```python
from build123d import *

# Parameters (mm, degrees)
F1_DEPTH = 10
F2_T     = -1
F3_R     = 15.4445915984
F4_DEPTH = 25


with BuildPart() as f1:
    # F0 (on Top) → F1 (new body)
    with BuildSketch(Plane.XY):
        Polygon((-24.2622910139, -14.8777581411), (-53.029731502, -60.6361962855), (54.0178157389, -60.6361962855), (22.2354376062, -14.8777581411), (48.3378368161, -14.8777581411), (10.1295774803, 33.7235331535), (24.2622910139, 33.7235331535), (0, 68.0067832147), (-24.2622910139, 33.7235331535), (-8.3033312269, 33.7235331535), (-47.1593588355, -14.8777581411), align=None)
    extrude(amount=F1_DEPTH)

    # F2
    f2_openings = [f1.faces().sort_by_distance(p)[0] for p in [
        (0.198833, -13.317224, 10),
    ]]
    offset(amount=F2_T, openings=f2_openings, kind=Kind.INTERSECTION)

    # F3 (on face) → F4 (cut)
    with BuildSketch(Plane.XY.offset(1)):
        Circle(F3_R)
    extrude(amount=-F4_DEPTH, mode=Mode.SUBTRACT)


solid = f1.part
```
Check sheet for the modelled part. Datum: model origin and axes. Units: mm. A direction names the side the tool comes from. Round coordinates to 2 decimals unless told otherwise and drop trailing zeros. Order: outer loops, then holes, each group sorted by start corner. A loop starts at its lowest first (then second) coordinate and runs counter-clockwise, first axis right, second up. Notation, with made-up numbers: (-18, 87.25) - (26, 87.25) arc R25 ccw to (26, 121.25) - close; hole circle Ø11 at (25, 28). An arc over 180 degrees is marked (long way). Answer as CSV lines item,"result". Start each with the question number.
1) Depth check by flat-ended pin: pin 1 (1 mm diameter, centred on y = -44, z = 7, fed in from +X); pin 2 (18.5 mm diameter, centred on x = 0, y = 0, fed in from -Z); pin 3 (4.5 mm diameter, centred on x = 16.5, z = 6, fed in from +Y); pin 4 (1.5 mm diameter, centred on y = 2.5, z = 4, fed in from -X). Enter the tip coordinate at first touch or a pass-through.
2) Tool access check on faces 1 (the face through (-11.01, 50.72, 5.44)), 2 (the face through (-36, -14.878, 5)), 3 (the face through (38.35, -38.08, 4.93)), 4 (the face through (-11.96, 51.11, 4.93)). Record the directions out of +Z, -Z, +X, -X, +Y, -Y that give a thin tool (end or side, any length) a straight path to the whole face; none if there is none.
3) Section check A-A (z = 7.75). Record the cut outline in (x, y), then the cut area to 3 significant figures.
4) Section check B-B (x = -17.5). Record the cut outline in (y, z), then the cut area to 3 significant figures.
5) Draft check along X on faces 5 (the face through (-16, 33.724, 5)), 6 (the face through (0, -59.636, 5)), 7 (the face through (-38.445, -37.437, 4.93)). Enter one of: +X half, -X half, draft (parallel to the pull), parting line (faces both ways), or undercut.
6) Scan lines: probe 1 along Y at (x, z) = (0, 0.8); probe 2 along Y at (x, z) = (-23, 9); probe 3 along Y at (x, z) = (27.5, 1.5). Record each from-to range of solid material in increasing order.
7) Section check C-C (y = -8). Record the cut outline in (x, z), then the cut area to 3 significant figures.
8) Section check D-D (y = 29). Record the cut outline in (x, z).
Determined:
1,pin 1,"x = 42.81"
1,pin 2,"through"
1,pin 3,"y = 47.87"
1,pin 4,"x = -33.87"
2,face 1,"+Z"
2,face 2,"+Z, -Z, -X"
2,face 3,"+Z, -Z, +X"
2,face 4,"+Z, -Z, -X, +Y"
3,outline,"(-53.03, -60.64) - (54.02, -60.64) - (22.24, -14.88) - (48.34, -14.88) - (10.13, 33.72) - (24.26, 33.72) - (0, 68.01) - (-24.26, 33.72) - (-8.3, 33.72) - (-47.16, -14.88) - (-24.26, -14.88) - close; hole (-51.22, -59.64) - (52.11, -59.64) - (20.32, -13.88) - (46.28, -13.88) - (8.07, 34.72) - (22.33, 34.72) - (0, 66.28) - (-22.33, 34.72) - (-6.22, 34.72) - (-45.08, -13.88) - (-22.45, -13.88) - close"
3,area,"499 mm^2"
4,outline,"(-60.64, 0) - (22.22, 0) - (22.22, 10) - (20.62, 10) - (20.62, 1) - (-59.64, 1) - (-59.64, 10) - (-60.64, 10) - close; (33.72, 0) - (43.28, 0) - (43.28, 10) - (41.55, 10) - (41.55, 1) - (34.72, 1) - (34.72, 10) - (33.72, 10) - close"
4,area,"140 mm^2"
5,face 5,"draft"
5,face 6,"undercut"
5,face 7,"-X half"
6,probe 1,"-60.64 to -15.44, 15.44 to 68.01"
6,probe 2,"-60.64 to -59.64, -14.75 to -13.88, 13.74 to 15.34, 33.72 to 35.51"
6,probe 3,"-60.64 to -59.64, -24.21 to -22.46, -14.88 to -13.88, 10.01 to 11.63"
7,outline,"(-41.66, 0) - (-13.21, 0) - (-13.21, 1) - (-40.38, 1) - (-40.38, 10) - (-41.66, 10) - close; (13.21, 0) - (42.93, 0) - (42.93, 10) - (41.66, 10) - (41.66, 1) - (13.21, 1) - close"
7,area,"81.1 mm^2"
8,outline,"(-12.08, 0) - (13.84, 0) - (13.84, 10) - (12.57, 10) - (12.57, 1) - (-10.8, 1) - (-10.8, 10) - (-12.08, 10) - close"
